Autodesk Inventor part; units mm, degrees
ref_plane "YZ Plane" through (0, 0, 0) normal (1, 0, 0) x (0, 1, 0)
ref_plane "XZ Plane" through (0, 0, 0) normal (0, 1, 0) x (-1, 0, 0)
ref_plane "XY Plane" through (0, 0, 0) normal (0, 0, 1) x (1, 0, 0)
sketch "BeltOuterProfile" plane through (0, 0, 0) normal (0, 0, 1) x (1, 0, 0)
  arc A0 (0, 34.2925) -> (0, -34.2925) centre (0, 0) ccw
  arc A1 (145, -34.2925) -> (145, 34.2925) centre (145, 0) ccw
  line L0 (0, 34.2925) -> (145, 34.2925)
  line L1 (0, -34.2925) -> (145, -34.2925)
  line L2 (0, 0) -> (500, 0) construction
  line L3 (145, 34.2925) -> (145, 0) construction
  line L4 (145, 0) -> (145, -34.2925) construction
  line L5 (0, 0) -> (0, 34.2925) construction
  line L6 (0, 0) -> (0, -34.2925) construction
  dimension "BeltLength" = 500
  dimension "CenterDistance" = 145
  dimension "d24" = 34.2925
  dimension "d25" = 34.2925
extrude "BeltWidth" add sketch "BeltOuterProfile" along normal blind 15
sketch "BeltThickness" plane through (0, 0, 15) normal (0, 0, 1) x (1, 0, 0)
  arc A0 (0, 34.2925) -> (0, -34.2925) centre (0, 0) ccw
  line L0 (0, -34.2925) -> (145, -34.2925)
  arc A1 (145, -34.2925) -> (145, 34.2925) centre (145, 0) ccw
  line L1 (145, 34.2925) -> (0, 34.2925)
  arc A2 (0, 30.4925) -> (0, -30.4925) centre (0, 0) ccw
  line L2 (0, -30.4925) -> (145, -30.4925)
  arc A3 (145, -30.4925) -> (145, 30.4925) centre (145, 0) ccw
  line L3 (145, 30.4925) -> (0, 30.4925)
  dimension "d17" = 3.8
extrude "BeltInternalAreaCut" cut sketch "BeltThickness" against normal through all contours L3 A3 L2 A2
equation "\"Pulley1WrapLength\" = 1"
equation "\"Pulley2WrapLength\" = 1"
properties part number "Belt Calculator" material "Nylon 6/6"
The model under review builds one solid part; all positions refer to its coordinate system, in mm. A direction names the side the tool comes from. Give positions to 0.01 mm unless a question says otherwise; leave off trailing zeros. Write each loop counter-clockwise with the first axis right and the second up, starting at its lowest first coordinate (ties: lowest second). Pieces come first, ordered by that corner, then holes.
1. Add section A-A, the plane x = 33. Write out the cut boundary in (y, z), plus the area to 3 significant figures.
2. Wall thickness on L1, parallel to Y at x = 42, z = 7.75; L2, parallel to X at y = -0.5, z = 7; L3, parallel to X at y = -23.5, z = 14: over which ranges is each line inside the solid? List them lowest first.
3. Tool access review of faces 1 (the flat face through (71, 34.292, 7)), 2 (the cylindrical face through (175.485, -0.671, 7.605)): name each direction out of +Z, -Z, +X, -X, +Y, -Y from which nothing blocks a thin tool from reaching the whole face with its end or side.
4. Add section C-C, the plane y = 0. Write out the cut boundary in (x, z), plus the area to 3 significant figures.
5. For P1, Ø8, axis at y = -19.5, z = 2, coming from the -X side; P2, Ø2, axis at y = 15, z = 10, coming from the +X side; P3, Ø6, axis at y = 16, z = 13, coming from the -X side, all flat-tipped, find the tip position at first contact; note any pin that passes through.
6. Draft analysis for pull direction Y (two halves, no side actions). For faces 3 (the cylindrical face through (-30.485, 0.671, 7.605)), 4 (the flat face through (71, -34.292, 7)), 5 (the cylindrical face through (179.284, 0.754, 7.395)), state which applies: +Y half, -Y half, draft (parallel to the pull), parting line (faces both ways), or undercut.
7. Add section B-B, the plane z = 8. Write out the cut boundary in (x, y) (1 decimal).
Worked answers:
1. outline: (-34.29, 0) - (-30.49, 0) - (-30.49, 15) - (-34.29, 15) - close; (30.49, 0) - (34.29, 0) - (34.29, 15) - (30.49, 15) - close
1. area: 114 mm2
2. L1: y = -34.29 to -30.49, 30.49 to 34.29
2. L2: x = -34.29 to -30.49, 175.49 to 179.29
2. L3: x = -24.97 to -19.43, 164.43 to 169.97
3. face 1: +Z, -Z, +X, -X, +Y
3. face 2: +Z, -Z
4. outline: (-34.29, 0) - (-30.49, 0) - (-30.49, 15) - (-34.29, 15) - close; (175.49, 0) - (179.29, 0) - (179.29, 15) - (175.49, 15) - close
4. area: 114 mm2
5. P1: stops at x = -30.59
5. P2: stops at x = 176.3
5. P3: stops at x = -31.73
6. face 3: undercut
6. face 4: -Y half
6. face 5: parting line
7. outline: (0, -34.3) - (145, -34.3) arc R34.3 ccw to (145, 34.3) - (0, 34.3) arc R34.3 ccw to start; hole (0, -30.5) - (145, -30.5) arc R30.5 ccw to (145, 30.5) - (0, 30.5) arc R30.5 ccw to start
